Can you work these out from the model? Positions are in its coordinate system, mm. Give positions to 0.01 mm unless a question says otherwise; leave off trailing zeros. Order: outer loops, then holes, each group sorted by start corner. A loop starts at its lowest first (then second) coordinate and runs counter-clockwise, first axis right, second up. Notation, with made-up numbers: (89, 64.25) - (129, 64.25) arc R17 ccw to (129, 76.25) - close; hole circle Ø7 at (-28.5, 80). An arc over 180 degrees is marked (long way). Answer as CSV lines item,"result".
```python
from build123d import *

# Parameters (mm, degrees)
SKETCH1_W                                  = 50.8
SKETCH1_H                                  = 50.8
BOSS_EXTRUDE1_DEPTH                        = 228.6
SKETCH2_W                                  = 8.89
SKETCH2_H                                  = 220.98
CUT_EXTRUDE1_DEPTH                         = 8.89
F_4_0_209_DIAMETER_HOLE1_D                 = 5.3086
F_4_0_209_DIAMETER_HOLE1_DEPTH             = 3.81
F_4_0_209_DIAMETER_HOLE2_D                 = 5.3086
MIRROR1_AT_THE_SECOND_PLANE_COPY_1_SKETC_W = 8.89
MIRROR1_AT_THE_SECOND_PLANE_COPY_1_SKETC_H = 220.98
MIRROR1_AT_THE_SECOND_PLANE_COPY_1_DEPTH   = 8.89
MIRROR1_AT_THE_SECOND_PLANE_COPY_2_D       = 5.3086
MIRROR1_AT_THE_SECOND_PLANE_COPY_2_DEPTH   = 3.81
MIRROR1_AT_THE_SECOND_PLANE_COPY_3_D       = 5.3086


with BuildPart() as part:
    # Sketch1 → Boss-Extrude1 (new body)
    with BuildSketch(Plane(origin=(0, 0, 0), x_dir=(1, 0, 0), z_dir=(0, 1, 0))):
        Rectangle(SKETCH1_W, SKETCH1_H)
    extrude(amount=BOSS_EXTRUDE1_DEPTH)

    # Sketch2 → Cut-Extrude1 (cut)
    with BuildSketch(Plane.XY.offset(25.4)):
        with Locations((20.955, 114.3)):
            Rectangle(SKETCH2_W, SKETCH2_H)
    cut_extrude1 = extrude(amount=-CUT_EXTRUDE1_DEPTH, mode=Mode.SUBTRACT)

    # #4 (0.209) Diameter Hole1
    with Locations(Plane(origin=(0, 3.81, 0), x_dir=(1, 0, 0), z_dir=(0, 1, 0))):
        with Locations((21.59, -21.59)):
            f_4_0_209_diameter_hole1 = Hole(F_4_0_209_DIAMETER_HOLE1_D / 2, depth=F_4_0_209_DIAMETER_HOLE1_DEPTH)

    # #4 (0.209) Diameter Hole2 (through all)
    with Locations(Plane(origin=(0, 224.79, 0), x_dir=(-1, 0, 0), z_dir=(0, -1, 0))):
        with Locations((-21.59, -21.59)):
            f_4_0_209_diameter_hole2 = Hole(F_4_0_209_DIAMETER_HOLE2_D / 2)

    # Mirror1: Cut-Extrude1, #4 (0.209) Diameter Hole1, #4 (0.209) Diameter Hole2 across plane
    add(cut_extrude1.mirror(Plane(origin=(0, 0, 0), x_dir=(0, 0, 1), z_dir=(1, 0, 0))), mode=Mode.SUBTRACT)
    add(f_4_0_209_diameter_hole1.mirror(Plane(origin=(0, 0, 0), x_dir=(0, 0, 1), z_dir=(1, 0, 0))), mode=Mode.SUBTRACT)
    add(f_4_0_209_diameter_hole2.mirror(Plane(origin=(0, 0, 0), x_dir=(0, 0, 1), z_dir=(1, 0, 0))), mode=Mode.SUBTRACT)

    # Mirror1 at the second plane: Cut-Extrude1, #4 (0.209) Diameter Hole1, #4 (0.209) Diameter Hole2 across plane
    add(cut_extrude1.mirror(Plane.XY), mode=Mode.SUBTRACT)
    add(f_4_0_209_diameter_hole1.mirror(Plane.XY), mode=Mode.SUBTRACT)
    add(f_4_0_209_diameter_hole2.mirror(Plane.XY), mode=Mode.SUBTRACT)

    # Mirror1 at the second plane copy 1 sketc → Mirror1 at the second plane copy 1 (cut)
    with BuildSketch(Plane(origin=(0, 0, -25.4), x_dir=(-1, 0, 0), z_dir=(0, 0, -1))):
        with Locations((20.955, 114.3)):
            Rectangle(MIRROR1_AT_THE_SECOND_PLANE_COPY_1_SKETC_W, MIRROR1_AT_THE_SECOND_PLANE_COPY_1_SKETC_H)
    extrude(amount=-MIRROR1_AT_THE_SECOND_PLANE_COPY_1_DEPTH, mode=Mode.SUBTRACT)

    # Mirror1 at the second plane copy 2
    with Locations(Plane(origin=(0, 3.81, 0), x_dir=(-1, 0, 0), z_dir=(0, 1, 0))):
        with Locations((21.59, -21.59)):
            Hole(MIRROR1_AT_THE_SECOND_PLANE_COPY_2_D / 2, depth=MIRROR1_AT_THE_SECOND_PLANE_COPY_2_DEPTH)

    # Mirror1 at the second plane copy 3 (through all)
    with Locations(Plane.XZ.offset(-224.79)):
        with Locations((-21.59, -21.59)):
            Hole(MIRROR1_AT_THE_SECOND_PLANE_COPY_3_D / 2)


solid = part.part
```
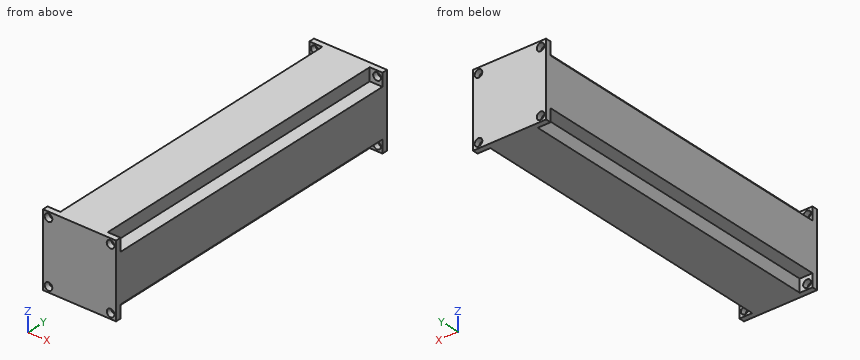
1) I'm going to push flat-ended pins straight in: P1, Ø3, axis at y = 145, z = -19.5, coming from the +X side; P2, Ø4.5, axis at y = 103, z = 22, coming from the -X side; P3, Ø5, axis at x = -21.59, z = 21.59, coming from the -Y side. Where does each tip first touch, or does it pass through?
Answer block:
P1,"x = 16.51"
P2,"x = -16.51"
P3,"through"
2) I want a section at B-B on x = -21.59. Write out the boundary of the cut face in (y, z), plus the area to 3 significant figures.
Answer block:
outline,"(0, -25.4) - (3.81, -25.4) - (3.81, -24.24) - (0, -24.24) - close; (0, -18.94) - (3.81, -18.94) - (3.81, -16.51) - (224.79, -16.51) - (224.79, -18.94) - (228.6, -18.94) - (228.6, 18.94) - (224.79, 18.94) - (224.79, 16.51) - (3.81, 16.51) - (3.81, 18.94) - (0, 18.94) - close; (0, 24.24) - (3.81, 24.24) - (3.81, 25.4) - (0, 25.4) - close; (224.79, -25.4) - (228.6, -25.4) - (228.6, -24.24) - (224.79, -24.24) - close; (224.79, 24.24) - (228.6, 24.24) - (228.6, 25.4) - (224.79, 25.4) - close"
area,"7,600 mm2"
3) I want a section at C-C on y = 121.5. Write out the boundary of the cut face in (x, z).
Answer block:
outline,"(-25.4, -16.51) - (-16.51, -16.51) - (-16.51, -25.4) - (16.51, -25.4) - (16.51, -16.51) - (25.4, -16.51) - (25.4, 16.51) - (16.51, 16.51) - (16.51, 25.4) - (-16.51, 25.4) - (-16.51, 16.51) - (-25.4, 16.51) - close"
4) I want a section at A-A on z = -21.59. Write out the boundary of the cut face in (x, y).
Answer block:
outline,"(-25.4, 0) - (-24.24, 0) - (-24.24, 3.81) - (-25.4, 3.81) - close; (-25.4, 224.79) - (-24.24, 224.79) - (-24.24, 228.6) - (-25.4, 228.6) - close; (-18.94, 0) - (18.94, 0) - (18.94, 3.81) - (16.51, 3.81) - (16.51, 224.79) - (18.94, 224.79) - (18.94, 228.6) - (-18.94, 228.6) - (-18.94, 224.79) - (-16.51, 224.79) - (-16.51, 3.81) - (-18.94, 3.81) - close; (24.24, 0) - (25.4, 0) - (25.4, 3.81) - (24.24, 3.81) - close; (24.24, 224.79) - (25.4, 224.79) - (25.4, 228.6) - (24.24, 228.6) - close"
5) I need wall thicknesses on line 1 along Z through (x, y) = (21.59, 227.8); line 2 along X through (y, z) = (2, -21). Which ranges of each line are inside material? Lowest first, please. Write a range as [from, to].
Answer block:
line 1,"[-25.4, -24.24], [-18.94, 18.94], [24.24, 25.4]"
line 2,"[-25.4, -24.18], [-19, 19], [24.18, 25.4]"
